```python
from build123d import *

# Parameters (mm, degrees)
ESQUISSE1_R        = 1.65
ESQUISSE1_R_2      = 1.603139346
ESQUISSE1_R_3      = 1.605
ESQUISSE1_R_4      = 4.25
ESQUISSE1_R_5      = 2
ESQUISSE1_W        = 50.4
ESQUISSE1_H        = 5.2
ESQUISSE1_W_2      = 5.4
ESQUISSE1_H_2      = 50.4
BOSS_EXTRU_1_DEPTH = 5


with BuildPart() as part:
    # Esquisse1 → Boss.-Extru.1 (new body)
    with BuildSketch(Plane.XY):
        Polygon((-220, 100), (-0.145812859, 100), (9.854187141, 100), (220, 100), (220, -100), (-220, -100), align=None)
        with Locations((-67.3, -94.376990981)):
            Circle(ESQUISSE1_R, mode=Mode.SUBTRACT)
        with Locations(Location((67.3, -94.376990981, 0), (0, 0, 180))):
            Circle(ESQUISSE1_R, mode=Mode.SUBTRACT)
        with Locations((152.3, -41.249056917)):
            Circle(ESQUISSE1_R_2, mode=Mode.SUBTRACT)
        with Locations((152.3, 28.750943083)):
            Circle(ESQUISSE1_R_3, mode=Mode.SUBTRACT)
        with Locations((67.3, 28.750943083)):
            Circle(ESQUISSE1_R_3, mode=Mode.SUBTRACT)
        with Locations((67.3, -41.249056917)):
            Circle(ESQUISSE1_R_3, mode=Mode.SUBTRACT)
        with Locations((-67.3, 28.750943083)):
            Circle(ESQUISSE1_R_3, mode=Mode.SUBTRACT)
        with Locations((-67.3, -41.249056917)):
            Circle(ESQUISSE1_R_3, mode=Mode.SUBTRACT)
        with Locations((-152.3, 28.750943083)):
            Circle(ESQUISSE1_R_3, mode=Mode.SUBTRACT)
        with Locations((-152.3, -41.249056917)):
            Circle(ESQUISSE1_R_3, mode=Mode.SUBTRACT)
        Circle(ESQUISSE1_R_4, mode=Mode.SUBTRACT)
        with Locations((0, -29.269007759)):
            Circle(ESQUISSE1_R_5, mode=Mode.SUBTRACT)
        with Locations((21.213203436, -38.055804324)):
            Circle(ESQUISSE1_R_5, mode=Mode.SUBTRACT)
        with Locations((30, -59.269007759)):
            Circle(ESQUISSE1_R_5, mode=Mode.SUBTRACT)
        with Locations((21.213203436, -80.482211195)):
            Circle(ESQUISSE1_R_5, mode=Mode.SUBTRACT)
        with Locations((0, -89.269007759)):
            Circle(ESQUISSE1_R_5, mode=Mode.SUBTRACT)
        with Locations((-21.213203436, -80.482211195)):
            Circle(ESQUISSE1_R_5, mode=Mode.SUBTRACT)
        with Locations((-30, -59.269007759)):
            Circle(ESQUISSE1_R_5, mode=Mode.SUBTRACT)
        with Locations((-21.213203436, -38.055804324)):
            Circle(ESQUISSE1_R_5, mode=Mode.SUBTRACT)
        with Locations((-49.8, 92.4)):
            Rectangle(ESQUISSE1_W, ESQUISSE1_H, mode=Mode.SUBTRACT)
        with Locations((-149.8, 92.4)):
            Rectangle(ESQUISSE1_W, ESQUISSE1_H, mode=Mode.SUBTRACT)
        with Locations((50.2, 92.4)):
            Rectangle(ESQUISSE1_W, ESQUISSE1_H, mode=Mode.SUBTRACT)
        with Locations((150.2, 92.4)):
            Rectangle(ESQUISSE1_W, ESQUISSE1_H, mode=Mode.SUBTRACT)
        with Locations((-212.3, -50.2)):
            Rectangle(ESQUISSE1_W_2, ESQUISSE1_H_2, mode=Mode.SUBTRACT)
        with Locations((-212.3, 29.8)):
            Rectangle(ESQUISSE1_W_2, ESQUISSE1_H_2, mode=Mode.SUBTRACT)
        with Locations((212.3, -50.2)):
            Rectangle(ESQUISSE1_W_2, ESQUISSE1_H_2, mode=Mode.SUBTRACT)
        with Locations((212.3, 29.8)):
            Rectangle(ESQUISSE1_W_2, ESQUISSE1_H_2, mode=Mode.SUBTRACT)
        with Locations((150.2, -92.4)):
            Rectangle(ESQUISSE1_W, ESQUISSE1_H, mode=Mode.SUBTRACT)
        with Locations((-149.8, -92.4)):
            Rectangle(ESQUISSE1_W, ESQUISSE1_H, mode=Mode.SUBTRACT)
    extrude(amount=BOSS_EXTRU_1_DEPTH)


solid = part.part
```
Source: CAD feature listing. Evaluate the final solid. Frame: model axes, mm. Coordinates: 2 decimals unless noted, no trailing zeros. Loops run counter-clockwise (first coordinate to the right, second up) from the corner with the lowest first, then second, coordinate; pieces in that order, holes last. Notation, with made-up numbers: M 45,55 L 54,55 A19 ccw 54,71 Z; hole C 62.25,-20.75 d8. An arc over 180 degrees is marked long. Use CSV: the item, a comma, the result in double quotes.
(1) Line query: line 1 (Y direction, x = 30, z = 3.4); line 2 (X direction, y = 45.5, z = 4.55); line 3 (Y direction, x = -174.5, z = 4). Output: solid intervals per line, ascending. Write a range as [from, to].
Answers follow:
line 1,"[-100, -61.27], [-57.27, 89.8], [95, 100]"
line 2,"[-220, -215], [-209.6, 209.6], [215, 220]"
line 3,"[-100, -95], [-89.8, 89.8], [95, 100]"
(2) Cut plane C-C on x = 41. Return loops of the section in (y, z), and give its area (3 significant figures).
Answers follow:
outline,"M -100,0 L 89.8,0 L 89.8,5 L -100,5 Z; M 95,0 L 100,0 L 100,5 L 95,5 Z"
area,"974 mm²"
(3) Cut plane A-A on y = -49. Return loops of the section in (x, z).
Answers follow:
outline,"M -220,0 L -215,0 L -215,5 L -220,5 Z; M -209.6,0 L 209.6,0 L 209.6,5 L -209.6,5 Z; M 215,0 L 220,0 L 220,5 L 215,5 Z"
(4) Cut plane B-B on y = 0. Return loops of the section in (x, z).
Answers follow:
outline,"M -220,0 L -4.25,0 L -4.25,5 L -220,5 Z; M 4.25,0 L 220,0 L 220,5 L 4.25,5 Z"
(5) Contact query for a flat-ended pin moving along its axis: pin 1 (6.5 mm diameter, centred on x = -30, y = -59.27, fed in from +Z). Output: stop coordinate, or through.
Answers follow:
pin 1,"z = 5"
(6) Cut plane D-D on x = -162. Return loops of the section in (y, z), and give its area (3 significant figures).
Answers follow:
outline,"M -100,0 L -95,0 L -95,5 L -100,5 Z; M -89.8,0 L 89.8,0 L 89.8,5 L -89.8,5 Z; M 95,0 L 100,0 L 100,5 L 95,5 Z"
area,"948 mm²"
(7) Draft query along Y for faces 1 (the face through (2.285, 3.584, 2.465)), 2 (the face through (3, -21, 5)). Return one class per face: pulls with the +Y half, pulls with the -Y half, needs draft (parallel to the pull), parting line crosses it, or undercut.
Answers follow:
face 1,"undercut"
face 2,"needs draft"
